```python
from build123d import *

# Parameters (mm, degrees)
SKETCH1_W                                    = 101.6
SKETCH1_H                                    = 57.15
BOSS_EXTRUDE1_DEPTH                          = 3.175
CSK_FOR_10_FLAT_HEAD_MACHINE_SCREW1_AT_COUNT = 2
CSK_FOR_10_FLAT_HEAD_MACHINE_SCREW1_AT_PITCH = 31.75
CSK_FOR_10_FLAT_HEAD_MACHINE_SCREW1_2_COUNT  = 2
CSK_FOR_10_FLAT_HEAD_MACHINE_SCREW1_2_PITCH  = 76.2
CSK_FOR_10_FLAT_HEAD_MACHINE_SCREW1_3_COUNT  = 2
CSK_FOR_10_FLAT_HEAD_MACHINE_SCREW1_3_PITCH  = 82.55


with BuildPart() as part:
    # Sketch1 → Boss-Extrude1 (new body)
    with BuildSketch(Plane(origin=(0, 0, 0), x_dir=(1, 0, 0), z_dir=(0, 1, 0))):
        Rectangle(SKETCH1_W, SKETCH1_H)
    extrude(amount=BOSS_EXTRUDE1_DEPTH)

    # Sketch10 → CSK for #10 Flat Head Machine Screw1 (revolve, cut)
    with BuildSketch(Plane(origin=(-38.1, 0, 15.875), x_dir=(0, 0, -1), z_dir=(1, 0, 0))):
        Polygon((0, 0), (0, 3.175), (2.5527, 3.175), (2.5527, 2.688180894), (4.8895, 0), align=None)
    csk_for_10_flat_head_machine_screw1 = revolve(axis=Axis((-38.1, -6.35, 15.875), (0, 1, 0)), mode=Mode.SUBTRACT)

    # CSK for #10 Flat Head Machine Screw1 at: CSK for #10 Flat Head Machine Screw1 ×2
    with Locations(*[(0, 0, -i * CSK_FOR_10_FLAT_HEAD_MACHINE_SCREW1_AT_PITCH) for i in range(1, CSK_FOR_10_FLAT_HEAD_MACHINE_SCREW1_AT_COUNT)]):
        add(csk_for_10_flat_head_machine_screw1, mode=Mode.SUBTRACT)

    # CSK for _10 Flat Head Machine Screw1 2: CSK for #10 Flat Head Machine Screw1 ×2
    with Locations(*[(i * CSK_FOR_10_FLAT_HEAD_MACHINE_SCREW1_2_PITCH, 0, 0) for i in range(1, CSK_FOR_10_FLAT_HEAD_MACHINE_SCREW1_2_COUNT)]):
        add(csk_for_10_flat_head_machine_screw1, mode=Mode.SUBTRACT)

    # CSK for _10 Flat Head Machine Screw1 3: CSK for #10 Flat Head Machine Screw1 ×2
    with Locations(*[Vector(0.9230769230769231, 0, -0.38461538461538464) * (i * CSK_FOR_10_FLAT_HEAD_MACHINE_SCREW1_3_PITCH) for i in range(1, CSK_FOR_10_FLAT_HEAD_MACHINE_SCREW1_3_COUNT)]):
        add(csk_for_10_flat_head_machine_screw1, mode=Mode.SUBTRACT)


solid = part.part
```
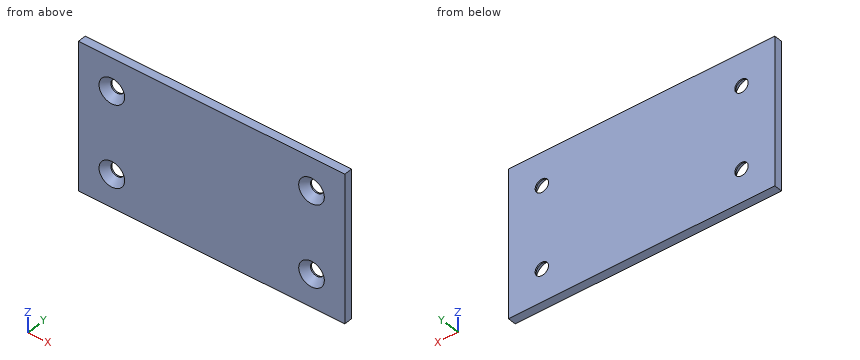
Can you work these out from the model? Positions are in its coordinate system, mm. Round coordinates to 2 decimals unless told otherwise and drop trailing zeros. Loops run counter-clockwise (first coordinate to the right, second up) from the corner with the lowest first, then second, coordinate; pieces in that order, holes last. Notation, with made-up numbers: (60.25, -21) -> (97.25, -21) arc R15 ccw to (97.25, -8) -> close; hole circle Ø6 at (-9, -20). An arc over 180 degrees is marked (long way). Answer in a Markdown table with one row per item.
Item 1: Will these pins go through, and if not, where does the flat tip stop? P1, Ø1.5, axis at x = 8, z = 19, coming from the -Y side; P2, Ø4.5, axis at x = 38.1, z = -15.875, coming from the -Y side.
Answer block:
| item | result |
|---|---|
| P1 | y = 0 |
| P2 | through |
Item 2: Suppose I cut it at B-B, the plane y = 0.6. List the corners of the cut face in (x, z) for me (3 decimals), plus the area to 3 significant figures.
Answer block:
| item | result |
|---|---|
| outline | (-50.8, -28.575) -> (50.8, -28.575) -> (50.8, 28.575) -> (-50.8, 28.575) -> close; hole circle Ø8.736 at (-38.1, -15.875); hole circle Ø8.736 at (-38.1, 15.875); hole circle Ø8.736 at (38.1, -15.875); hole circle Ø8.736 at (38.1, 15.875) |
| area | 5,570 mm² |
Item 3: If I drill on probe 1 along Z at (x, y) = (38.1, 2.8) (3 decimals); probe 2 along X at (y, z) = (2.8, 16); probe 3 along X at (y, z) = (1.65, -19), over which ranges is the centre line in solid material (lowest first)?
Answer block:
| item | result |
|---|---|
| probe 1 | -28.575 to -18.428, -13.322 to 13.322, 18.428 to 28.575 |
| probe 2 | -50.8 to -40.65, -35.55 to 35.55, 40.65 to 50.8 |
| probe 3 | -50.8 to -39.57, -36.63 to 36.63, 39.57 to 50.8 |
Item 4: Suppose I cut it at A-A, the plane x = 38.1. List the corners of the cut face in (y, z) for me (1 decimal), plus the area to 3 significant figures.
Answer block:
| item | result |
|---|---|
| outline | (0, -28.6) -> (3.2, -28.6) -> (3.2, -18.4) -> (2.7, -18.4) -> (0, -20.8) -> close; (0, -11) -> (2.7, -13.3) -> (3.2, -13.3) -> (3.2, 13.3) -> (2.7, 13.3) -> (0, 11) -> close; (0, 20.8) -> (2.7, 18.4) -> (3.2, 18.4) -> (3.2, 28.6) -> (0, 28.6) -> close |
| area | 136 mm² |
